from build123d import *

# Parameters (mm, degrees)
F0_W      = 92.96126
F0_H      = 63.60507
F1_DEPTH  = 50.8
F4_R      = 5.08
F5_R      = 5.08
F6_R      = 5.08
F7_W      = 7
F7_H      = 14
F8_DEPTH  = 16
F9_W      = 7
F9_H      = 14
F10_DEPTH = 16
F11_W     = 6.9
F11_H     = 1.85
F12_DEPTH = 16


with BuildPart() as f1:
    # F0 (on Front) → F1 (new body)
    with BuildSketch(Plane.XZ):
        Rectangle(F0_W, F0_H)
    extrude(amount=F1_DEPTH)

    # F4
    f4_edges = [f1.edges().sort_by_distance(p)[0] for p in [
        (0, -50.8, 31.802535),
    ]]
    fillet(f4_edges, radius=F4_R)

    # F5
    f5_edges = [f1.edges().sort_by_distance(p)[0] for p in [
        (0, 0, 31.802535),
    ]]
    fillet(f5_edges, radius=F5_R)

    # F6
    f6_edges = [f1.edges().sort_by_distance(p)[0] for p in [
        (0, -50.8, -31.802535),
        (0, 0, -31.802535),
    ]]
    fillet(f6_edges, radius=F6_R)

    # F7 (on face) → F8 (cut)
    with BuildSketch(Plane.YZ.offset(46.48063)):
        with Locations((-42.770251, 21.441529)):
            Rectangle(F7_W, F7_H)
    extrude(amount=-F8_DEPTH, mode=Mode.SUBTRACT)

    # F9 (on face) → F10 (cut)
    with BuildSketch(Plane.YZ.offset(46.48063)):
        with Locations((-33.1692, 21.429915)):
            Rectangle(F9_W, F9_H)
    extrude(amount=-F10_DEPTH, mode=Mode.SUBTRACT)

    # F11 (on face) → F12 (cut)
    with BuildSketch(Plane.YZ.offset(46.48063)):
        with Locations((-21.729334, 24.124714)):
            Rectangle(F11_W, F11_H)
        with Locations((-21.445199, 16.760846)):
            Rectangle(F11_W, F11_H)
    extrude(amount=-F12_DEPTH, mode=Mode.SUBTRACT)


solid = f1.part
Geometry: final body of the model. Coordinates: model frame, mm. A direction names the side the tool comes from. Round coordinates to 2 decimals unless told otherwise and drop trailing zeros. Loops run counter-clockwise (first coordinate to the right, second up) from the corner with the lowest first, then second, coordinate; pieces in that order, holes last.
Q1. Access query for faces 1 (the cylindrical face through (0.651, -1.528, 30.354)), 2 (the flat face through (39, -22, 25.05)). Directions: +Z, -Z, +X, -X, +Y, -Y. A direction counts if a zero-diameter tool reaches every point of the face in a straight line with its end or side. Return the directions, or none.
Q2. Section A-A on y = -31.5. Return loops of the section in (x, z), plus the area to 3 significant figures.
Q3. Pin query (flat end, axial travel): P1, Ø0.6, axis at y = -23.5, z = 24.5, coming from the +X side; P2, Ø2, axis at y = -23, z = 16.5, coming from the +X side. Return the tip coordinate at first contact, or that it passes through.
Q4. Material intervals for L1, parallel to Z at x = 33.5, y = -34.5; L2, parallel to X at y = -22, z = 24; L3, parallel to Z at x = 28, y = -4.5, sorted ascending.
Q5. Pull-direction query (Y, two-part tool) for faces 3 (the flat face through (39, -33, 28.43)), 4 (the cylindrical face through (0.651, -49.272, 30.354)), 5 (the flat face through (39, -22, 23.2)), 6 (the flat face through (46.481, -25, 0)); classes: released by +Y, released by -Y, zero draft, split by the parting line, or undercut.
Evaluation:
1. face 1: +Z, +X, -X, +Y
1. face 2: +X
2. outline: (-46.48, -31.8) - (46.48, -31.8) - (46.48, 14.43) - (30.48, 14.43) - (30.48, 28.43) - (46.48, 28.43) - (46.48, 31.8) - (-46.48, 31.8) - close
2. area: 5,690 mm2
3. P1: stops at x = 30.48
3. P2: stops at x = 46.48
4. L1: z = -31.8 to 14.43, 28.43 to 31.8
4. L2: x = -46.48 to 30.48
4. L3: z = -31.77 to 31.77
5. face 3: undercut
5. face 4: released by -Y
5. face 5: undercut
5. face 6: zero draft
